Part model, mm, in its own coordinate system. A direction names the side the tool comes from. Coordinates: 2 decimals unless noted, no trailing zeros. Order: outer loops, then holes, each group sorted by start corner. A loop starts at its lowest first (then second) coordinate and runs counter-clockwise, first axis right, second up. Notation, with made-up numbers: M -1,50.5 L 33,50.5 A23 ccw 33,66.5 Z; hole C -5.5,12.5 d3. An arc over 180 degrees is marked long. Answer in a Markdown table with one row per item. Add a question column.
from build123d import *

# Parameters (mm, degrees)
F0_R      = 34.925
F1_DEPTH  = 825.5
F2_R      = 31.75
F3_DEPTH  = 69.85
F4_R      = 31.75
F5_DEPTH  = 101.6
F6_W      = 31.75
F6_H      = 31.75
F7_DEPTH  = 38.1
F8_R      = 25.4
F9_DEPTH  = 25.4
F10_R     = 31.75
F10_R_2   = 25.4
F11_DEPTH = 34.925
F14_DEPTH = 6.35


# Not quite as in the source:
# - a fillet or chamfer that OpenCascade refuses, or shapes differently, is made with other operations: its cross-section is extruded or revolved along the edge and cut away or added


with BuildPart() as f1:
    # F0 (on Front) → F1 (new body, symmetric)
    with BuildSketch(Plane.XZ):
        Circle(F0_R)
    extrude(amount=F1_DEPTH, both=True)

    # F2 (on face) → F3 (join)
    with BuildSketch(Plane.XZ.offset(825.5)):
        Circle(F2_R)
    extrude(amount=F3_DEPTH)

    # F4 (on face) → F5 (join)
    with BuildSketch(Plane(origin=(0, 825.5, 0), x_dir=(-1, 0, 0), z_dir=(0, 1, 0))):
        Circle(F4_R)
    extrude(amount=F5_DEPTH)

    # F6 (on face) → F7 (join)
    with BuildSketch(Plane.XZ.offset(895.35)):
        Rectangle(F6_W, F6_H)
    extrude(amount=F7_DEPTH)

    # F8 (on face) → F9 (join)
    with BuildSketch(Plane(origin=(0, 927.1, 0), x_dir=(-1, 0, 0), z_dir=(0, 1, 0))):
        Circle(F8_R)
    extrude(amount=F9_DEPTH)

    # F10 (on face) → F11 (join)
    with BuildSketch(Plane(origin=(0, 952.5, 0), x_dir=(-1, 0, 0), z_dir=(0, 1, 0))):
        Circle(F10_R)
        Circle(F10_R_2, mode=Mode.SUBTRACT)
        Circle(F10_R_2)
    extrude(amount=F11_DEPTH)

    # F12: fillet of radius 5.08 on 4 edges, made by hand

    # F12_s1 → F12_t2 (revolve, cut)
    with BuildSketch(Plane.XY):
        with BuildLine():
            ThreePointArc((31.75, 825.5), (34.0571134838, 823.6305202921), (34.925, 820.7907139607))
            Line((34.925, 820.7907139607), (34.925, 825.5))
            Line((34.925, 825.5), (31.75, 825.5))
        make_face()
    revolve(axis=Axis((0, 825.5, 0), (0, -1, 0)), mode=Mode.SUBTRACT)

    # F12_s3 → F12_t4 (revolve, cut)
    with BuildSketch(Plane.XY):
        with BuildLine():
            ThreePointArc((34.925, -820.7907139607), (34.0571134838, -823.6305202921), (31.75, -825.5))
            Line((31.75, -825.5), (34.925, -825.5))
            Line((34.925, -825.5), (34.925, -820.7907139607))
        make_face()
    revolve(axis=Axis((0, -825.5, 0), (0, -1, 0)), mode=Mode.SUBTRACT)

    # F12_s5 → F12_t6 (revolve, cut)
    with BuildSketch(Plane.XY):
        with BuildLine():
            ThreePointArc((31.75, -890.27), (30.2621024484, -893.8621024484), (26.67, -895.35))
            Line((26.67, -895.35), (31.75, -895.35))
            Line((31.75, -895.35), (31.75, -890.27))
        make_face()
    revolve(axis=Axis((0, -895.35, 0), (0, -1, 0)), mode=Mode.SUBTRACT)

    # F12_s7 → F12_t8 (revolve, cut)
    with BuildSketch(Plane.XY):
        with BuildLine():
            ThreePointArc((-26.67, 927.1), (-30.2621024484, 925.6121024484), (-31.75, 922.02))
            Line((-31.75, 922.02), (-31.75, 927.1))
            Line((-31.75, 927.1), (-26.67, 927.1))
        make_face()
    revolve(axis=Axis((0, 927.1, 0), (0, 1, 0)), mode=Mode.SUBTRACT)

    # F13 (on face) → F14 (cut)
    with BuildSketch(Plane(origin=(0, 987.425, 0), x_dir=(-1, 0, 0), z_dir=(0, 1, 0))):
        Polygon((2.749630657, 4.7625), (-2.749630657, 4.7625), (-5.499261314, 0), (-2.749630657, -4.7625), (2.749630657, -4.7625), (5.499261314, 0), align=None)
    extrude(amount=-F14_DEPTH, mode=Mode.SUBTRACT)


solid = f1.part
(1) Slice it at A-A (y = 867). List the corners of the cut face in (x, z).
(2) Pull direction Y, two halves, no side cores. Call faces 1 (the flat face through (0, -933.45, 0)), 2 (the flat face through (-24, 927.1, -10)), 3 (the cylindrical face through (5.506, 939.622, -24.796)), 4 (the flat face through (-15.875, -914, 0)): pulls with the +Y half, pulls with the -Y half, needs draft (parallel to the pull), parting line crosses it, or undercut.
(3) Slice it at B-B (y = 1). List the corners of the cut face in (x, z) (3 decimals), and give its area (3 significant figures).
(4) Drop flat-ended pins along their axis: P1, Ø4.5, axis at x = 0, y = 985, coming from the +Z side; P2, Ø10, axis at y = 544.5, z = -6.5, coming from the +X side; P3, Ø16, axis at x = 7.5, y = -920.5, coming from the +Z side (3 decimals). Give the stop position or say it passes through.
(5) 3-axis set-ups, long thin cutter, end or side, ignore diameter. For faces 5 (the cylindrical face through (-6.883, -857.432, -30.995)), 6 (the flat face through (0, -914, 15.875)), 7 (the flat face through (15.875, -914, 0)): which of +Z, -Z, +X, -X, +Y, -Y reach the whole face in a straight line?
(6) Wall check: line 1 (Y direction, x = 24.5, z = 13) (3 decimals); line 2 (Y direction, x = -9, z = 18.5) (3 decimals); line 3 (Y direction, x = -26.5, z = -9) (3 decimals). Give the ranges that are in metal, low to high.
Computed:
| question | item | result |
|---|---|---|
| 1 | outline | C 0,0 d63.5 |
| 2 | face 1 | pulls with the -Y half |
| 2 | face 2 | undercut |
| 2 | face 3 | undercut |
| 2 | face 4 | needs draft |
| 3 | outline | C 0,0 d69.85 |
| 3 | area | 3,830 mm^2 |
| 4 | P1 | stops at z = 31.75 |
| 4 | P2 | stops at x = 34.89 |
| 4 | P3 | stops at z = 15.875 |
| 5 | face 5 | -Y |
| 5 | face 6 | +Z, +X, -X, -Y |
| 5 | face 7 | +Z, -Z, +X, -Y |
| 6 | line 1 | y = -895.237 to 926.987, 952.5 to 987.425 |
| 6 | line 2 | y = -895.35 to 987.425 |
| 6 | line 3 | y = -895.176 to 926.926, 952.5 to 987.425 |
